from build123d import *

# Parameters (mm, degrees)
SKETCH2_W               = 250
SKETCH2_H               = 80
BOSS_EXTRUDE1_DEPTH     = 30
SKETCH11_R              = 6
CUT_EXTRUDE2_DEPTH      = 265.196896272
CUT_EXTRUDE_THIN2_DEPTH = 265.196896272
SKETCH15_W              = 40
SKETCH15_H              = 20
CUT_EXTRUDE3_DEPTH      = 25
SKETCH16_R              = 12.5
BOSS_EXTRUDE2_DEPTH     = 50


with BuildPart() as part:
    # Sketch2 → Boss-Extrude1 (new body)
    with BuildSketch(Plane(origin=(0, 0, 0), x_dir=(0, 0, -1), z_dir=(1, 0, 0))):
        with Locations((125, 40)):
            Rectangle(SKETCH2_W, SKETCH2_H)
    extrude(amount=BOSS_EXTRUDE1_DEPTH)

    # Sketch11 → Cut-Extrude2 (cut, through all)
    with BuildSketch(Plane(origin=(30, 0, 0), x_dir=(0, 0, -1), z_dir=(1, 0, 0))):
        with Locations((40, 40)):
            Circle(SKETCH11_R)
    extrude(amount=-CUT_EXTRUDE2_DEPTH, mode=Mode.SUBTRACT)

    # Sketch14 → Cut-Extrude-Thin2 (cut, through all)
    with BuildSketch(Plane.ZY):
        with BuildLine():
            ThreePointArc((-40, 0), (0, 40), (-40, 80))
            Line((-40, 80), (-40, 90))
            ThreePointArc((-40, 90), (10, 40), (-40, -10))
            Line((-40, -10), (-40, 0))
        make_face()
        with BuildLine():
            ThreePointArc((-210, 80), (-250, 40), (-210, 0))
            Line((-210, 0), (-210, -10))
            ThreePointArc((-210, -10), (-260, 40), (-210, 90))
            Line((-210, 90), (-210, 80))
        make_face()
    extrude(amount=-CUT_EXTRUDE_THIN2_DEPTH, mode=Mode.SUBTRACT)


with BuildPart() as cut_extrude_thin2_kept_piece:
    # of the separate pieces the step leaves, the one the design keeps (cut_extrude_thin2_pieces_kept)
    add(part.part.solids().sort_by_distance((0, 0, -40))[0])

    # Sketch15 → Cut-Extrude3 (cut)
    with BuildSketch(Plane.ZY):
        with Locations((-210, 40)):
            Rectangle(SKETCH15_W, SKETCH15_H)
    extrude(amount=-CUT_EXTRUDE3_DEPTH, mode=Mode.SUBTRACT)

    # Sketch16 → Boss-Extrude2 (add)
    with BuildSketch(Plane(origin=(0, 0, -230), x_dir=(-1, 0, 0), z_dir=(0, 0, -1))):
        with Locations(Location((-15, 40, 0), (0, 0, 180))):
            Circle(SKETCH16_R)
    extrude(amount=BOSS_EXTRUDE2_DEPTH)


solid = cut_extrude_thin2_kept_piece.part
Model file for the job. Use its own axes, mm. A direction names the side the tool comes from. Coordinates: 2 decimals unless noted, no trailing zeros. Loops run counter-clockwise (first coordinate to the right, second up) from the corner with the lowest first, then second, coordinate; pieces in that order, holes last. Notation, with made-up numbers: (61, 25.5) -> (81, 25.5) arc R27 ccw to (81, 63.5) -> close; hole circle Ø11 at (66, -5). An arc over 180 degrees is marked (long way). Use one line per item in the form item = value. Start each with the question number.
(1) Cut at C-C on z = -239. Give the cut face in (x, y).
(2) Cut at B-B on x = 18.5. Give the cut face in (y, z), and give its area (3 significant figures).
(3) Pull direction Z, two halves, no side cores. Call faces 3 (the cylindrical face through (14.79, 54.5, -247.28)), 4 (the cylindrical face through (2.512, 39.45, -263.774)), 5 (the flat face through (12, 50, -210)), 6 (the cylindrical face through (14.79, 39.12, -0.01)): pulls with the +Z half, pulls with the -Z half, needs draft (parallel to the pull), parting line crosses it, or undercut.
(4) Probe probe 1 along Y at (x, z) = (13, -40); probe 2 along Y at (x, z) = (22.5, -206.5); probe 3 along Z at (x, y) = (5, 43). List the from-to ranges inside material, lowest first. Write a range as from..to.
(5) Cut at A-A on y = 40. Give the cut face in (x, z), and give its area (3 significant figures).
(6) Flat gauge pins, fed straight in: pin 1 (3 mm diameter, centred on x = 19, y = 61, fed in from +Z); pin 2 (12 mm diameter, centred on x = 22, y = 67, fed in from -Z); pin 3 (16 mm diameter, centred on x = 18.5, y = 38, fed in from +Z). Where does each tip first touch, or does it go through?
(7) Cut at D-D on y = 8. Give the cut face in (x, z).
(8) Tool access for faces 1 (the flat face through (12, 40, -230)), 2 (the flat face through (0, 41, -123)): list every direction of +Z, -Z, +X, -X, +Y, -Y with a clear straight run to the whole face (end or side of a thin tool).
Values:
q1.outline = (0, 12.45) -> (30, 12.45) -> (30, 67.55) -> (0, 67.55) -> close
q2.outline = (0, -210) arc R40 ccw to (28, -248.16) -> (28, -280) -> (52, -280) -> (52, -248.16) arc R40 ccw to (80, -210) -> (80, -40) arc R40 ccw to (0, -40) -> close; hole (30, -230) -> (50, -230) -> (50, -190) -> (30, -190) -> close; hole circle Ø12 at (40, -40)
q2.area = 18,400 mm2
q3.face_3 = pulls with the -Z half
q3.face_4 = needs draft
q3.face_5 = undercut
q3.face_6 = pulls with the +Z half
q4.probe_1 = 0..34, 46..80
q4.probe_2 = 0..30, 50..80
q4.probe_3 = -280..-230, -190..-45.2, -34.8..-0.11
q5.outline = (0, -250) -> (2.5, -250) -> (2.5, -280) -> (27.5, -280) -> (27.5, -250) -> (30, -250) -> (30, -46) -> (0, -46) -> (0, -190) -> (25, -190) -> (25, -230) -> (0, -230) -> close; (0, -34) -> (30, -34) -> (30, 0) -> (0, 0) -> close
q5.area = 6,890 mm2
q6.pin_1 = -5.08
q6.pin_2 = -244.04
q6.pin_3 = 0
q7.outline = (0, -234) -> (30, -234) -> (30, -16) -> (0, -16) -> close
q8.face_1 = -X
q8.face_2 = +Z, -Z, -X, +Y, -Y
